Source: CAD feature listing. Evaluate the final solid. Frame: model axes, mm. A direction names the side the tool comes from. Give positions to 0.01 mm unless a question says otherwise; leave off trailing zeros. Order: outer loops, then holes, each group sorted by start corner. A loop starts at its lowest first (then second) coordinate and runs counter-clockwise, first axis right, second up.
```python
from build123d import *

# Parameters (mm, degrees)
EXTRUDE_1_DEPTH              = 11.5
CUT_EXTRUDE_1_DEPTH          = 5
CUT_EXTRUDE_2_DEPTH          = 5
HOLE_WIZARD_3_0_3_1_D        = 3
HOLE_WIZARD_3_0_3_2_D        = 3
HOLE_WIZARD_2_5_2_5_1_REACH  = 21.112
HOLE_WIZARD_2_5_2_5_1_BORE_R = 1.25
HOLE_WIZARD_5_0_5_1_D        = 5
HOLE_WIZARD_6_0_6_1_D        = 6
HOLE_WIZARD_2_5_2_5_2_REACH  = 21.112
HOLE_WIZARD_2_5_2_5_2_BORE_R = 1.25
CHAMFER_1_SIZE               = 3


with BuildPart() as part:
    # Эскиз1 → Бобышка-Вытянуть1 (new body)
    with BuildSketch(Plane(origin=(0, 0, 0), x_dir=(-1, 0, 0), z_dir=(0, 0, -1))):
        with BuildLine():
            Line((6.75, 8), (-9.75, 8))
            ThreePointArc((-9.75, 8), (-13, 0), (-9.75, -8))
            Line((-9.75, -8), (6.75, -8))
            ThreePointArc((6.75, -8), (10, 0), (6.75, 8))
        make_face()
    extrude(amount=-EXTRUDE_1_DEPTH)

    # Эскиз2 → Вырез-Вытянуть1 (cut)
    with BuildSketch(Plane(origin=(0, 0, 0), x_dir=(-1, 0, 0), z_dir=(0, 0, -1))):
        with BuildLine():
            Line((-4, 6), (8.305725542, 6))
            ThreePointArc((8.305725542, 6), (7.583253924, 7.043086716), (6.75, 8))
            Line((6.75, 8), (-4, 8))
            Line((-4, 8), (-4, 6))
        make_face()
    extrude(amount=-CUT_EXTRUDE_1_DEPTH, mode=Mode.SUBTRACT)

    # Эскиз3 → Вырез-Вытянуть2 (cut)
    with BuildSketch(Plane(origin=(0, 0, 0), x_dir=(-1, 0, 0), z_dir=(0, 0, -1))):
        with BuildLine():
            Line((8.305725542, -6), (-4, -6))
            Line((-4, -6), (-4, -8))
            Line((-4, -8), (6.75, -8))
            ThreePointArc((6.75, -8), (7.583253924, -7.043086716), (8.305725542, -6))
        make_face()
    extrude(amount=-CUT_EXTRUDE_2_DEPTH, mode=Mode.SUBTRACT)

    # Диаметр отверстия Ø3.0 (3)1 (through all)
    with Locations(Plane.XY.offset(11.5)):
        with Locations((0, -6), (0, 6)):
            Hole(HOLE_WIZARD_3_0_3_1_D / 2)

    # Диаметр отверстия Ø3.0 (3)2 (through all)
    with Locations(Plane(origin=(0, 8, 0), x_dir=(1, 0, 0), z_dir=(0, 1, 0))):
        with Locations((-5, -7)):
            Hole(HOLE_WIZARD_3_0_3_2_D / 2)

    # Диаметр отверстия Ø2.5 (2.5)1 bore → Диаметр отверстия Ø2.5 (2.5)1 (cut, up to next)
    with BuildSketch(Plane(origin=(0, 0, 0), x_dir=(-1, 0, 0), z_dir=(0, 0, -1)), mode=Mode.PRIVATE) as hole_wizard_2_5_2_5_1_sk1:
        with Locations((5, 0)):
            Circle(HOLE_WIZARD_2_5_2_5_1_BORE_R)
    hole_wizard_2_5_2_5_1_tool1 = extrude(hole_wizard_2_5_2_5_1_sk1.sketch, amount=-HOLE_WIZARD_2_5_2_5_1_REACH, mode=Mode.PRIVATE) & part.part
    add(hole_wizard_2_5_2_5_1_tool1.solids().sort_by_distance((-5, 0, 0))[0], mode=Mode.SUBTRACT)

    # Диаметр отверстия Ø5.0 (5)1 (through all)
    with Locations(Plane(origin=(0, 0, 0), x_dir=(-1, 0, 0), z_dir=(0, 0, -1))):
        with Locations((0, 0)):
            Hole(HOLE_WIZARD_5_0_5_1_D / 2)

    # Диаметр отверстия Ø6.0 (6)1 (through all)
    with Locations(Plane(origin=(0, -8, 0), x_dir=(-1, 0, 0), z_dir=(0, -1, 0))):
        with Locations((-7, -7.25)):
            Hole(HOLE_WIZARD_6_0_6_1_D / 2)

    # Диаметр отверстия Ø2.5 (2.5)2 bore → Диаметр отверстия Ø2.5 (2.5)2 (cut, up to next)
    with BuildSketch(Plane(origin=(0, 0, 0), x_dir=(-1, 0, 0), z_dir=(0, 0, -1)), mode=Mode.PRIVATE) as hole_wizard_2_5_2_5_2_sk1:
        with Locations((-7, 0)):
            Circle(HOLE_WIZARD_2_5_2_5_2_BORE_R)
    hole_wizard_2_5_2_5_2_tool1 = extrude(hole_wizard_2_5_2_5_2_sk1.sketch, amount=-HOLE_WIZARD_2_5_2_5_2_REACH, mode=Mode.PRIVATE) & part.part
    add(hole_wizard_2_5_2_5_2_tool1.solids().sort_by_distance((7, 0, 0))[0], mode=Mode.SUBTRACT)

    # Фаска1
    chamfer_1_edges = [part.edges().sort_by_distance(p)[0] for p in [
        (-10, 0, 0),
        (13, 0, 0),
    ]]
    chamfer(chamfer_1_edges, length=CHAMFER_1_SIZE)


solid = part.part
```
1) Section query D-D, the plane z = 9. Return the cut outline in (x, y), and give its area (3 significant figures).
Report:
outline: (-6.75, -8) - (4.56, -8) - (4.56, 8) - (-6.75, 8) arc R11.47 ccw to start; (9.44, -8) - (9.75, -8) arc R11.47 ccw to (9.75, 8) - (9.44, 8) - close; hole circle Ø5 at (0, 0); hole circle Ø3 at (0, -6); hole circle Ø3 at (0, 6)
area: 224 mm2
2) Pin query (flat end, axial travel): pin 1 (0.6 mm diameter, centred on y = -7, z = 1.5, fed in from -X); pin 2 (2 mm diameter, centred on y = 3.5, z = 3.5, fed in from -X); pin 3 (2 mm diameter, centred on x = 7, y = 0, fed in from -Z); pin 4 (0.6 mm diameter, centred on x = -0.5, y = -6.5, fed in from -Z). Return the tip coordinate at first contact, or that it passes through.
Report:
pin 1: stops at x = 4
pin 2: stops at x = -9.72
pin 3: stops at z = 10.08
pin 4: passes through
3) Draft query along Z for faces 4 (the cylindrical face through (8.384, 0.112, 9.912)), 5 (the flat face through (4, 7, 2)), 6 (the flat face through (4, 0, 0)), 7 (the cylindrical face through (-5.69, -0.11, 8.33)). Return one class per face: +Z half, -Z half, draft (parallel to the pull), parting line (faces both ways), or undercut.
Report:
face 4: undercut
face 5: draft
face 6: -Z half
face 7: undercut
4) Section query C-C, the plane x = 0. Return the cut outline in (y, z), and give its area (3 significant figures).
Report:
outline: (-8, 5) - (-7.5, 5) - (-7.5, 11.5) - (-8, 11.5) - close; (-4.5, 0) - (-2.5, 0) - (-2.5, 11.5) - (-4.5, 11.5) - close; (2.5, 0) - (4.5, 0) - (4.5, 11.5) - (2.5, 11.5) - close; (7.5, 5) - (8, 5) - (8, 11.5) - (7.5, 11.5) - close
area: 52.5 mm2
5) Section query A-A, the plane y = 0. Return the cut outline in (x, z), and give its area (3 significant figures).
Report:
outline: (-10, 3) - (-7, 0) - (-6.25, 0) - (-6.25, 6.17) arc R1.5 cw (long way) to (-3.75, 6.17) - (-3.75, 0) - (-2.5, 0) - (-2.5, 11.5) - (-10, 11.5) - close; (2.5, 0) - (5.75, 0) - (5.75, 4.52) arc R3 cw (long way) to (8.25, 4.52) - (8.25, 0) - (10, 0) - (13, 3) - (13, 11.5) - (2.5, 11.5) - close
area: 138 mm2
6) Reachability of faces 1 (the flat face through (3, -6, 2)), 2 (the flat face through (2, -8, 7)), 3 (the flat face through (-4, 6, 3)) from +Z, -Z, +X, -X, +Y, -Y: full face, straight path, thin tool, end or side. Return the list, or none.
Report:
face 1: -Z, -X, -Y
face 2: +Z, -Z, +X, -X, -Y
face 3: -Z, -X, +Y
7) Material intervals for L1, parallel to Y at x = 0, z = 6; L2, parallel to Z at x = 7, y = 3.5; L3, parallel to Y at x = 1, z = 9.25, sorted ascending.
Report:
L1: y = -8 to -7.5, -4.5 to -2.5, 2.5 to 4.5, 7.5 to 8
L2: z = 0 to 4.25, 10.25 to 11.5
L3: y = -8 to -7.12, -4.88 to -2.29, 2.29 to 4.88, 7.12 to 8
8) Section query B-B, the plane z = 7.25. Return the cut outline in (x, y), and give its area (3 significant figures).
Report:
outline: (-6.75, -8) - (-6.48, -8) - (-6.48, 8) - (-6.75, 8) arc R11.47 ccw to start; (-3.52, -8) - (4, -8) - (4, 8) - (-3.52, 8) - close; (10, -7.73) arc R11.47 ccw to (10, 7.73) - close; hole circle Ø5 at (0, 0); hole circle Ø3 at (0, -6); hole circle Ø3 at (0, 6)
area: 159 mm2
